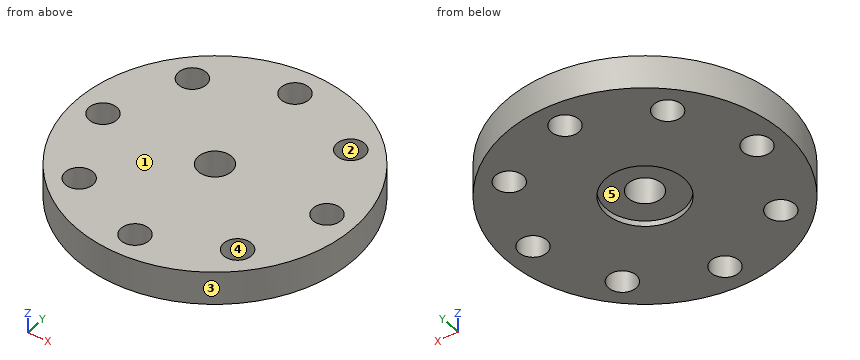
```python
from build123d import *

# Parameters (mm, degrees)
SKETCH1_R           = 12.5
SKETCH1_R_2         = 1.25
SKETCH1_R_3         = 1.5
BOSS_EXTRUDE1_DEPTH = 3
SKETCH3_R           = 3.5
SKETCH3_R_2         = 1.5
CUT_EXTRUDE1_DEPTH  = 0.5


with BuildPart() as part:
    # Sketch1 → Boss-Extrude1 (new body)
    with BuildSketch(Plane.XY):
        Circle(SKETCH1_R)
        with Locations((0, 10)):
            Circle(SKETCH1_R_2, mode=Mode.SUBTRACT)
        Circle(SKETCH1_R_3, mode=Mode.SUBTRACT)
        with Locations((7.071067812, 7.071067812)):
            Circle(SKETCH1_R_2, mode=Mode.SUBTRACT)
        with Locations((10, 0)):
            Circle(SKETCH1_R_2, mode=Mode.SUBTRACT)
        with Locations((7.071067812, -7.071067812)):
            Circle(SKETCH1_R_2, mode=Mode.SUBTRACT)
        with Locations((0, -10)):
            Circle(SKETCH1_R_2, mode=Mode.SUBTRACT)
        with Locations((-7.071067812, -7.071067812)):
            Circle(SKETCH1_R_2, mode=Mode.SUBTRACT)
        with Locations((-10, 0)):
            Circle(SKETCH1_R_2, mode=Mode.SUBTRACT)
        with Locations((-7.071067812, 7.071067812)):
            Circle(SKETCH1_R_2, mode=Mode.SUBTRACT)
    extrude(amount=BOSS_EXTRUDE1_DEPTH)

    # Sketch3 → Cut-Extrude1 (cut)
    with BuildSketch(Plane(origin=(0, 0, 0), x_dir=(-1, 0, 0), z_dir=(0, 0, -1))):
        Circle(SKETCH3_R)
        Circle(SKETCH3_R_2, mode=Mode.SUBTRACT)
    extrude(amount=-CUT_EXTRUDE1_DEPTH, mode=Mode.SUBTRACT)


solid = part.part
```
Geometry check sheet. Reference: the model listing, model coordinates, mm. Face numbers are marked on the shaded views. A direction names the side the tool comes from. Give positions to 0.01 mm unless a question says otherwise; leave off trailing zeros. Order: outer loops, then holes, each group sorted by start corner. A loop starts at its lowest first (then second) coordinate and runs counter-clockwise, first axis right, second up.
1. Section check B-B, the plane y = 0. Enter the section's corners in (x, z).
2. Thickness scan on L1, parallel to Y at x = 0, z = 1.35; L2, parallel to Y at x = 0, z = 0.15; L3, parallel to X at y = -6.5, z = 2.05. Record the ranges inside material, lowest first.
3. Section check D-D, the plane y = -7.5. Enter the section's corners in (x, z), and give its area (3 significant figures).
4. Section check A-A, the plane x = -10. Enter the section's corners in (y, z), and give its area (3 significant figures).
5. Access from +Z, -Z, +X, -X, +Y, -Y to the whole of each face (thin tool, end or side, straight path). Record for the marked faces 4 and 5.
6. Gauge pin test, flat end, axial feed: pin 1 Ø5.5 at (x, y) = (0, 0) entering from -Z. Record the tip position at first contact, or that the pin passes through.
7. Release check for a two-part mould opening along Y. For the marked faces 1, 2 and 3 record: pulls with the +Y half, pulls with the -Y half, needs draft (parallel to the pull), parting line crosses it, or undercut.
Values follow:
1. outline: (-12.5, 0) - (-11.25, 0) - (-11.25, 3) - (-12.5, 3) - close; (-8.75, 0) - (-3.5, 0) - (-3.5, 0.5) - (-1.5, 0.5) - (-1.5, 3) - (-8.75, 3) - close; (1.5, 0.5) - (3.5, 0.5) - (3.5, 0) - (8.75, 0) - (8.75, 3) - (1.5, 3) - close; (11.25, 0) - (12.5, 0) - (12.5, 3) - (11.25, 3) - close
2. L1: y = -12.5 to -11.25, -8.75 to -1.5, 1.5 to 8.75, 11.25 to 12.5
2. L2: y = -12.5 to -11.25, -8.75 to -3.5, 3.5 to 8.75, 11.25 to 12.5
2. L3: x = -10.68 to -8.18, -5.96 to 5.96, 8.18 to 10.68
3. outline: (-10, 0) - (-8.25, 0) - (-8.25, 3) - (-10, 3) - close; (-5.9, 0) - (5.9, 0) - (5.9, 3) - (-5.9, 3) - close; (8.25, 0) - (10, 0) - (10, 3) - (8.25, 3) - close
3. area: 45.9 mm2
4. outline: (-7.5, 0) - (-1.25, 0) - (-1.25, 3) - (-7.5, 3) - close; (1.25, 0) - (7.5, 0) - (7.5, 3) - (1.25, 3) - close
4. area: 37.5 mm2
5. face 4: +Z, -Z
5. face 5: -Z
6. pin 1: stops at z = 0.5
7. face 1: needs draft
7. face 2: undercut
7. face 3: parting line crosses it
